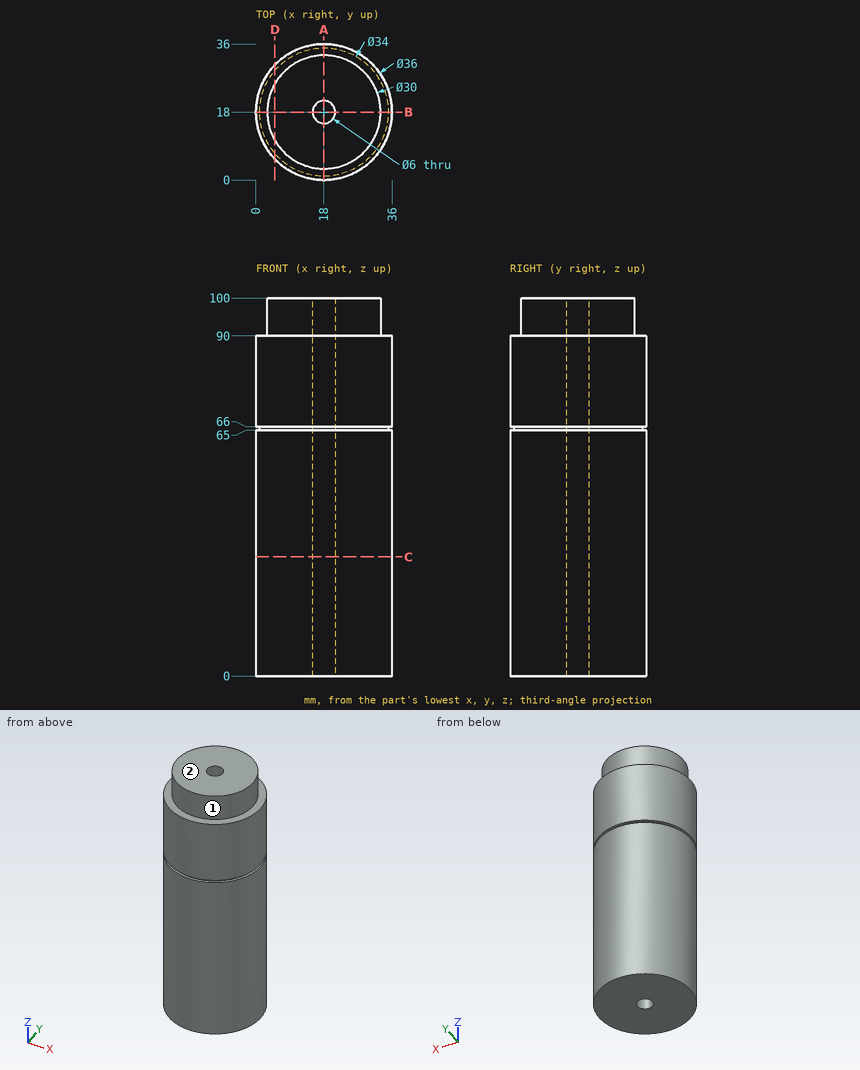
Could you check a few things on this drawing? It's one solid part, dimensions in mm from its lowest x, y, z. A direction names the side the tool comes from. Round coordinates to 2 decimals unless told otherwise and drop trailing zeros. Write each loop counter-clockwise with the first axis right and the second up, starting at its lowest first coordinate (ties: lowest second). Pieces come first, ordered by that corner, then holes.
Q1. Will these pins go through, and if not, where does the flat tip stop? P1, Ø3, axis at x = 4, z = 85.5, coming from the +Y side; P2, Ø6, axis at x = 24.5, z = 77.5, coming from the +Y side; P3, Ø4, axis at y = 25, z = 32, coming from the -X side.
Q2. If we section it at D-D on x = 5: Write out the boundary of the cut face in (y, z).
Q3. Please list where these lines run through material, in increasing order: probe 1 along Y at (x, z) = (18, 79.5); probe 2 along Z at (x, y) = (25.5, 32); probe 3 along X at (y, z) = (14, 40.5).
Q4. If we section it at A-A on x = 18: Write out the boundary of the cut face in (y, z), plus the area to 3 significant figures.
Q5. Which directions (+Z, -Z, +X, -X, +Y, -Y) give clear straight access to the entire face, cutting with the end or side of a thin tool? Please do the marked faces 1 and 2.
Q6. If we section it at C-C on z = 31.5: Write out the boundary of the cut face in (x, y).
Answer below:
1. P1: stops at y = 30.95
1. P2: stops at y = 35.66
1. P3: stops at x = 0.71
2. outline: (5.55, 0) - (30.45, 0) - (30.45, 65) - (28.95, 65) - (28.95, 66) - (30.45, 66) - (30.45, 90) - (25.48, 90) - (25.48, 100) - (10.52, 100) - (10.52, 90) - (5.55, 90) - (5.55, 66) - (7.05, 66) - (7.05, 65) - (5.55, 65) - close
3. probe 1: y = 0 to 15, 21 to 36
3. probe 2: z = 0 to 90
3. probe 3: x = 0.45 to 35.55
4. outline: (0, 0) - (15, 0) - (15, 100) - (3, 100) - (3, 90) - (0, 90) - (0, 66) - (1, 66) - (1, 65) - (0, 65) - close; (21, 0) - (36, 0) - (36, 65) - (35, 65) - (35, 66) - (36, 66) - (36, 90) - (33, 90) - (33, 100) - (21, 100) - close
4. area: 2,940 mm2
5. face 1: +Z
5. face 2: +Z, +X, -X, +Y, -Y
6. outline: circle Ø36 at (18, 18); hole circle Ø6 at (18, 18)
